Build history of the part. All positions in model axes, mm. A direction names the side the tool comes from. Give positions to 0.01 mm unless a question says otherwise; leave off trailing zeros. Order: outer loops, then holes, each group sorted by start corner. A loop starts at its lowest first (then second) coordinate and runs counter-clockwise, first axis right, second up. Notation, with made-up numbers: M -35,26 L 0,26 A7 cw 0,32 Z; hole C 74,41.25 d5. An arc over 180 degrees is marked long. One line per item, written item: value.
from build123d import *

# Parameters (mm, degrees)
SKETCH1_R           = 0.9
SKETCH1_W           = 4.2
SKETCH1_H           = 8
SKETCH1_W_2         = 8.2
SKETCH1_H_2         = 6
BOSS_EXTRUDE1_DEPTH = 2


with BuildPart() as part:
    # Sketch1 → Boss-Extrude1 (new body)
    with BuildSketch(Plane.XY):
        with BuildLine():
            Line((16.2, 109.64), (0, 109.64))
            Line((0, 109.64), (0, 99.66))
            ThreePointArc((0, 99.66), (0.585786438, 98.245786438), (2, 97.66))
            Line((2, 97.66), (2.75, 97.66))
            Line((2.75, 97.66), (2.75, 91.66))
            Line((2.75, 91.66), (2, 91.66))
            ThreePointArc((2, 91.66), (0.585786438, 91.074213562), (0, 89.66))
            Line((0, 89.66), (0, 69.21))
            ThreePointArc((0, 69.21), (0.585786438, 67.795786438), (2, 67.21))
            Line((2, 67.21), (4, 67.21))
            Line((4, 67.21), (4, 59.21))
            Line((4, 59.21), (2, 59.21))
            ThreePointArc((2, 59.21), (0.585786438, 58.624213562), (0, 57.21))
            Line((0, 57.21), (0, 28))
            ThreePointArc((0, 28), (0.585786438, 26.585786438), (2, 26))
            Line((2, 26), (4, 26))
            Line((4, 26), (4, 14))
            Line((4, 14), (6, 14))
            Line((6, 14), (6, 26))
            Line((6, 26), (10.2, 26))
            Line((10.2, 26), (10.2, 14))
            Line((10.2, 14), (12.2, 14))
            Line((12.2, 14), (12.2, 26))
            Line((12.2, 26), (14.2, 26))
            ThreePointArc((14.2, 26), (15.614213562, 26.585786438), (16.2, 28))
            Line((16.2, 28), (16.2, 57.21))
            ThreePointArc((16.2, 57.21), (15.614213562, 58.624213562), (14.2, 59.21))
            Line((14.2, 59.21), (12.2, 59.21))
            Line((12.2, 59.21), (12.2, 67.21))
            Line((12.2, 67.21), (14.2, 67.21))
            ThreePointArc((14.2, 67.21), (15.614213562, 67.795786438), (16.2, 69.21))
            Line((16.2, 69.21), (16.2, 89.66))
            ThreePointArc((16.2, 89.66), (15.614213562, 91.074213562), (14.2, 91.66))
            Line((14.2, 91.66), (13.45, 91.66))
            Line((13.45, 91.66), (13.45, 97.66))
            Line((13.45, 97.66), (14.2, 97.66))
            ThreePointArc((14.2, 97.66), (15.614213562, 98.245786438), (16.2, 99.66))
            Line((16.2, 99.66), (16.2, 109.64))
        make_face()
        with Locations((13.45, 56.71)):
            Circle(SKETCH1_R, mode=Mode.SUBTRACT)
        with Locations((10.2, 49.71)):
            Circle(SKETCH1_R, mode=Mode.SUBTRACT)
        with Locations((13.45, 106.16)):
            Circle(SKETCH1_R, mode=Mode.SUBTRACT)
        with Locations((2.75, 99.66)):
            Circle(SKETCH1_R, mode=Mode.SUBTRACT)
        with Locations((6, 49.71)):
            Circle(SKETCH1_R, mode=Mode.SUBTRACT)
        with Locations((2.75, 28.5)):
            Circle(SKETCH1_R, mode=Mode.SUBTRACT)
        with Locations((2.75, 89.16)):
            Circle(SKETCH1_R, mode=Mode.SUBTRACT)
        with Locations((2.75, 56.71)):
            Circle(SKETCH1_R, mode=Mode.SUBTRACT)
        with Locations((13.45, 89.16)):
            Circle(SKETCH1_R, mode=Mode.SUBTRACT)
        with Locations((13.45, 99.66)):
            Circle(SKETCH1_R, mode=Mode.SUBTRACT)
        with Locations((13.45, 69.71)):
            Circle(SKETCH1_R, mode=Mode.SUBTRACT)
        with Locations((6, 35.5)):
            Circle(SKETCH1_R, mode=Mode.SUBTRACT)
        with Locations((2.75, 106.16)):
            Circle(SKETCH1_R, mode=Mode.SUBTRACT)
        with Locations((10.2, 35.5)):
            Circle(SKETCH1_R, mode=Mode.SUBTRACT)
        with Locations((2.75, 69.71)):
            Circle(SKETCH1_R, mode=Mode.SUBTRACT)
        with Locations((13.45, 28.5)):
            Circle(SKETCH1_R, mode=Mode.SUBTRACT)
        with Locations((8.1, 63.21)):
            Rectangle(SKETCH1_W, SKETCH1_H, mode=Mode.SUBTRACT)
        with Locations((8.1, 94.66)):
            Rectangle(SKETCH1_W_2, SKETCH1_H_2, mode=Mode.SUBTRACT)
    extrude(amount=BOSS_EXTRUDE1_DEPTH)


solid = part.part
1) Saw through at C-C, the plane z = 1.55. Give the number of separate pieces and of enclosed holes in the cut face, then the cut area to 3 significant figures.
Check values:
separate pieces: 1
enclosed holes: 18
area: 1,170 mm^2
2) Saw through at B-B, the plane y = 106.16. Write the cut outline in (x, z).
Check values:
outline: M 0,0 L 1.85,0 L 1.85,2 L 0,2 Z; M 3.65,0 L 12.55,0 L 12.55,2 L 3.65,2 Z; M 14.35,0 L 16.2,0 L 16.2,2 L 14.35,2 Z
3) Tool access for faces 4 (the face through (4, 20, 1)), 5 (the face through (6, 20, 1)), 6 (the face through (12, 62, 2)), 7 (the face through (10.2, 63, 1)), 8 (the face through (15.6, 67.78, 0.99)): list every direction of +Z, -Z, +X, -X, +Y, -Y with a clear straight run to the whole face (end or side of a thin tool).
Check values:
face 4: +Z, -Z, -X, -Y
face 5: +Z, -Z, -Y
face 6: +Z, +X, -X, +Y, -Y
face 7: +Z, -Z
face 8: +Z, -Z, +X
4) Mould opens along Y. For faces 1 (the face through (8, 26, 1)), 2 (the face through (0, 105, 1)), 3 (the face through (13.45, 95, 1)) say: released by +Y, released by -Y, zero draft, split by the parting line, or undercut.
Check values:
face 1: released by -Y
face 2: zero draft
face 3: undercut
5) Drill centre lines: probe 1 along Y at (x, z) = (7, 1.3); probe 2 along X at (y, z) = (89, 1.7); probe 3 along X at (y, z) = (49.71, 1.3). Where is each one in solid material? Low to high. Write a range as from..to.
Check values:
probe 1: 26..59.21, 67.21..91.66, 97.66..109.64
probe 2: 0..1.86, 3.64..12.56, 14.34..16.2
probe 3: 0..5.1, 6.9..9.3, 11.1..16.2
6) Saw through at A-A, the plane y = 93. Write the cut outline in (x, z).
Check values:
outline: M 2.75,0 L 4,0 L 4,2 L 2.75,2 Z; M 12.2,0 L 13.45,0 L 13.45,2 L 12.2,2 Z
7) Pin check, flat tips, straight feed: pin 1 (3 mm diameter, centred on x = 13.45, y = 89.16, fed in from -Z); pin 2 (1 mm diameter, centred on x = 13.5, z = 1.5, fed in from -Y); pin 3 (1 mm diameter, centred on y = 65, z = 1, fed in from -X). Stop position of each tip, or through.
Check values:
pin 1: z = 0
pin 2: y = 26
pin 3: x = 4
